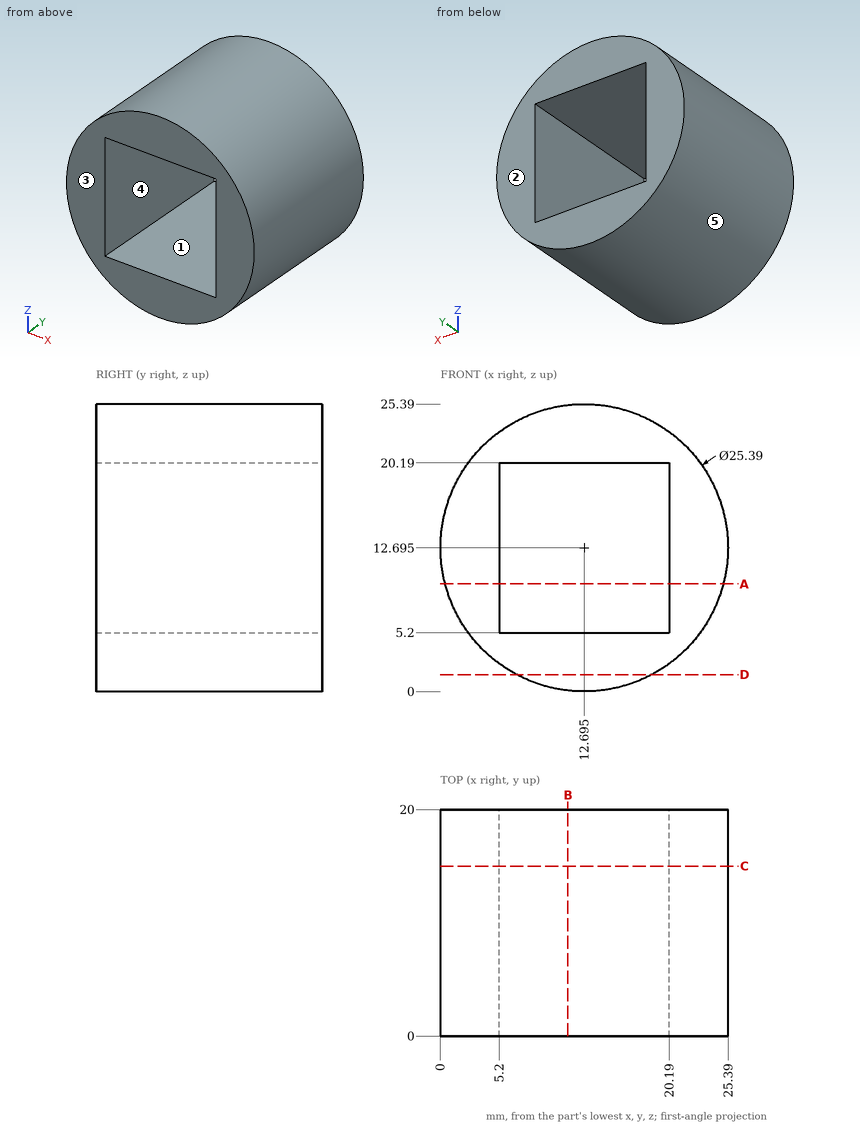
Input: dimensioned drawing with shaded views. Units: mm. Origin: part minimum x, y, z. A direction names the side the tool comes from. Give positions to 0.01 mm unless a question says otherwise; leave off trailing zeros. Order: outer loops, then holes, each group sorted by start corner. A loop starts at its lowest first (then second) coordinate and runs counter-clockwise, first axis right, second up. Notation, with made-up numbers: (55.25, 72.5) -> (81.25, 72.5) arc R18 ccw to (81.25, 89.5) -> close; hole circle Ø8 at (15.25, 12.25). An arc over 180 degrees is marked (long way). Use one line per item in the form item = value.
1) Section A-A, the plane z = 9.5. Return loops of the section in (x, y).
Response values:
outline = (0.41, 0) -> (5.2, 0) -> (5.2, 20) -> (0.41, 20) -> close; (20.19, 0) -> (24.98, 0) -> (24.98, 20) -> (20.19, 20) -> close
2) Mould query, pull axis Z, two halves, no side actions, for the marked faces 3, 4 and 5. Classes: pulls with the +Z half, pulls with the -Z half, needs draft (parallel to the pull), parting line crosses it, or undercut.
Response values:
face_3 = needs draft
face_4 = undercut
face_5 = parting line crosses it
3) Section B-B, the plane x = 11.25. Return loops of the section in (y, z), and give its area (3 significant figures).
Response values:
outline = (0, 0.08) -> (20, 0.08) -> (20, 5.2) -> (0, 5.2) -> close; (0, 20.19) -> (20, 20.19) -> (20, 25.31) -> (0, 25.31) -> close
area = 205 mm^2
4) Section C-C, the plane y = 15. Return loops of the section in (x, z) (3 decimals), and give its area (3 significant figures).
Response values:
outline = circle Ø25.39 at (12.695, 12.695); hole (5.2, 5.2) -> (20.19, 5.2) -> (20.19, 20.19) -> (5.2, 20.19) -> close
area = 282 mm^2
5) First-contact query: pin 1 Ø3 at (x, y) = (11, 16) entering from -Z; pin 2 Ø10 at (y, z) = (12.5, 7) entering from +X; pin 3 Ø2 at (y, z) = (10, 10.5) entering from -X; pin 4 Ø6 at (y, z) = (13.5, 20.5) entering from +X. Flat tips, straight axial feed; report the tip coordinate or a pass-through.
Response values:
pin_1 = 0
pin_2 = 25.37
pin_3 = 0.06
pin_4 = 24.45
6) Section D-D, the plane z = 1.5. Return loops of the section in (x, y).
Response values:
outline = (6.71, 0) -> (18.68, 0) -> (18.68, 20) -> (6.71, 20) -> close
7) Reachability of the marked faces 1 and 2 from +Z, -Z, +X, -X, +Y, -Y: full face, straight path, thin tool, end or side. Return the list, or none.
Response values:
face_1 = +Y, -Y
face_2 = +Z, -Z, +X, -X, +Y
8) Line query: probe 1 along X at (y, z) = (6.75, 13); probe 2 along X at (y, z) = (3.5, 8.75); probe 3 along Z at (x, y) = (19.75, 18.75). Output: solid intervals per line, ascending.
Response values:
probe_1 = 0 to 5.2, 20.19 to 25.39
probe_2 = 0.63 to 5.2, 20.19 to 24.76
probe_3 = 2.14 to 5.2, 20.19 to 23.25
